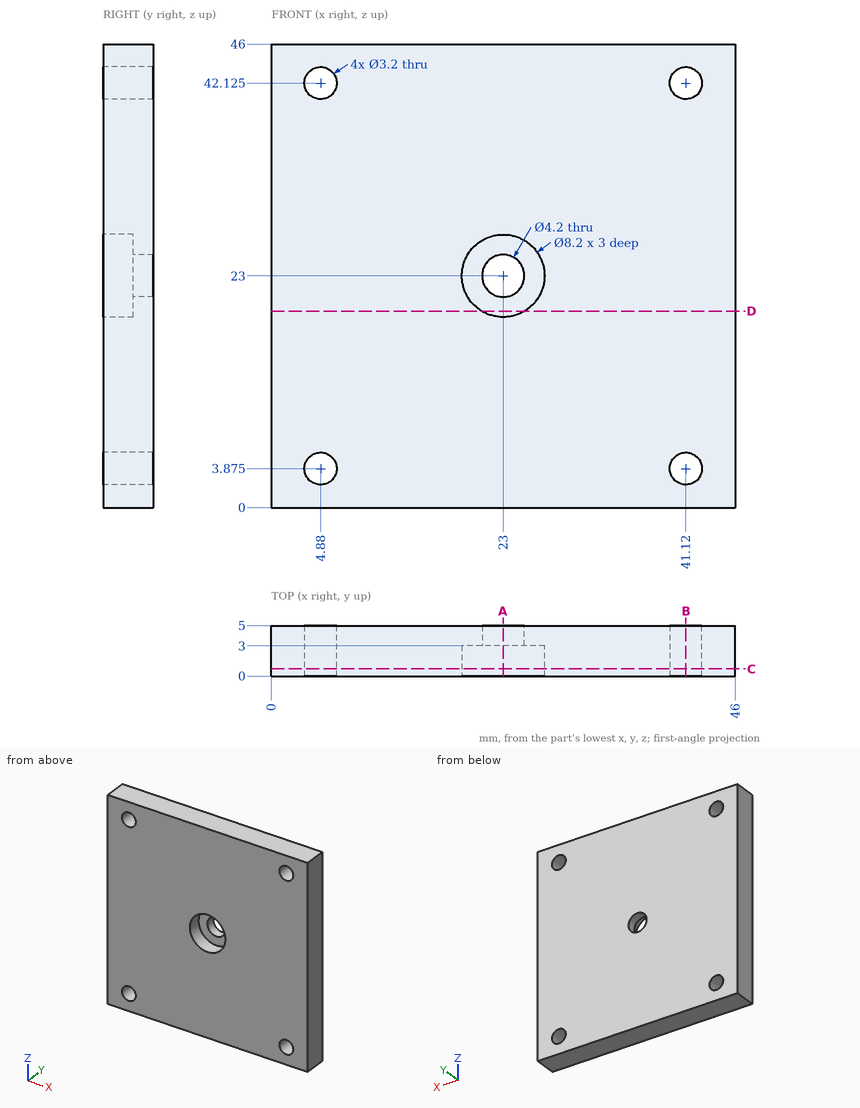
Design review of the part shown in the three views and the two pictorial views. Dimensions are in mm from the part's minimum x, y and z. Give positions to 0.01 mm unless a question says otherwise; leave off trailing zeros. Loops run counter-clockwise (first coordinate to the right, second up) from the corner with the lowest first, then second, coordinate; pieces in that order, holes last. Notation, with made-up numbers: (-5.5, -21) -> (-0.5, -21) arc R29 ccw to (-0.5, 0) -> close; hole circle Ø4 at (-35.5, -8.75). An arc over 180 degrees is marked (long way). Answer as a JSON object with one key per item and string values. Group by question number.
Q1. Take a section at C-C (y = 0.7). Write out the cut boundary in (x, z) (3 decimals).
Q2. Take a section at B-B (x = 41.12). Write out the cut boundary in (y, z) (3 decimals).
Q3. Insertion check: pin 1 (1.9 mm diameter, centred on x = 4.88, z = 42.125, fed in from +Y). The pin has a flat end and moves straight along its axis. Give the tip position at first contact, or say it passes through.
Q4. Take a section at D-D (z = 19.5). Write out the cut boundary in (x, y).
Q5. Wall thickness on line 1 along Z through (x, y) = (4.88, 2.8) (3 decimals); line 2 along X through (y, z) = (0.35, 41.5); line 3 along X through (y, z) = (0.4, 5): over which ranges is each line inside the solid? List them lowest first.
Q6. Take a section at A-A (x = 23). Write out the cut boundary in (y, z).
Answer below:
{
 "1": {"outline": "(0, 0) -> (46, 0) -> (46, 46) -> (0, 46) -> close; hole circle Ø3.2 at (4.88, 3.875); hole circle Ø3.2 at (4.88, 42.125); hole circle Ø8.2 at (23, 23); hole circle Ø3.2 at (41.12, 3.875); hole circle Ø3.2 at (41.12, 42.125)"},
 "2": {"outline": "(0, 0) -> (5, 0) -> (5, 2.275) -> (0, 2.275) -> close; (0, 5.475) -> (5, 5.475) -> (5, 40.525) -> (0, 40.525) -> close; (0, 43.725) -> (5, 43.725) -> (5, 46) -> (0, 46) -> close"},
 "3": {"pin 1": "passes through"},
 "4": {"outline": "(0, 0) -> (20.86, 0) -> (20.86, 3) -> (25.14, 3) -> (25.14, 0) -> (46, 0) -> (46, 5) -> (0, 5) -> close"},
 "5": {"line 1": "z = 0 to 2.275, 5.475 to 40.525, 43.725 to 46", "line 2": "x = 0 to 3.41, 6.35 to 39.65, 42.59 to 46", "line 3": "x = 0 to 3.74, 6.02 to 39.98, 42.26 to 46"},
 "6": {"outline": "(0, 0) -> (5, 0) -> (5, 20.9) -> (3, 20.9) -> (3, 18.9) -> (0, 18.9) -> close; (0, 27.1) -> (3, 27.1) -> (3, 25.1) -> (5, 25.1) -> (5, 46) -> (0, 46) -> close"}
}
